Input: part model. Units: mm. Frame: model coordinates. Face numbers are marked on the shaded views. Coordinates: 2 decimals unless noted, no trailing zeros. Write each loop counter-clockwise with the first axis right and the second up, starting at its lowest first coordinate (ties: lowest second). Pieces come first, ordered by that corner, then holes. Notation, with made-up numbers: (65.25, 18) - (105.25, 18) arc R21 cw to (105.25, 39) - close; hole circle Ø7 at (-0.75, 36). An arc over 180 degrees is marked (long way). One line per question, with ' | ' between items. Start each with the question number.
1) First-contact query: P1, Ø2, axis at x = 8.5, y = 5, coming from the -Z side; P2, Ø5, axis at x = -27, y = 3.5, coming from the +Z side; P3, Ø3.5, axis at x = -19.5, z = -16, coming from the -Y side. Flat tips, straight axial feed; report the tip coordinate or a pass-through.
2) Section query C-C on y = 4. Return loops of the section in (x, z).
3) Section query D-D on x = -16.5. Return loops of the section in (y, z).
4) Line query: line 1 (Z direction, x = 12, y = 3.25); line 2 (Y direction, x = 11.5, z = -16); line 3 (Z direction, x = 12.5, y = 7). Output: solid intervals per line, ascending.
5) Draft query along Z for the marked faces 1 and 2. Return one class per face: released by +Z, released by -Z, zero draft, split by the parting line, or undercut.
6) Section query A-A on x = 34.5. Return loops of the section in (y, z) (3 decimals), and give its area (3 significant figures).
7) Section query B-B on z = 0. Return loops of the section in (x, y).
Autodesk Inventor part; units mm, degrees
ref_plane "YZ Plane" through (0, 0, 0) normal (1, 0, 0) x (0, 1, 0)
ref_plane "XZ Plane" through (0, 0, 0) normal (0, 1, 0) x (-1, 0, 0)
ref_plane "XY Plane" through (0, 0, 0) normal (0, 0, 1) x (1, 0, 0)
sketch "Base Pattern" plane through (0, 0, 0) normal (0, 1, 0) x (-1, 0, 0)
  line L0 (50, 13.5) -> (-50, 13.5)
  line L1 (-50, 13.5) -> (-50, -13.5)
  line L2 (-50, -13.5) -> (50, -13.5)
  line L3 (50, -13.5) -> (50, 13.5)
  line L4 (50, 13.5) -> (-50, -13.5) construction
  line L5 (-50, 13.5) -> (50, -13.5) construction
  point P0 (0, 0)
  dimension "Length" = 100
  dimension "Base_Width" = 27
sketch "Slot Pattern Set-Out" plane through (0, 0, 0) normal (0, 1, 0) x (-1, 0, 0)
  line L0 (0, -25) -> (0, 25)
  line L1 (10.385, 2.115) -> (-10.385, 2.115)
  line L2 (-10.385, -2.115) -> (10.385, -2.115)
  arc A0 (10.385, -2.115) -> (10.385, 2.115) centre (10.385, 0) ccw
  arc A1 (-10.385, 2.115) -> (-10.385, -2.115) centre (-10.385, 0) ccw
  line L3 (32, 0) -> (-32, 0) construction
  line L4 (10.385, 0) -> (-10.385, 0) construction
  point P0 (0, 0)
  point P1 (0, 0)
  point P2 (0, 0)
  point P3 (0, 0)
  dimension "Slot_Length" = 20.77
  dimension "Slot_Dia" = 4.23
  dimension "Pattern_Length" = 64
extrude "Plate1" add sketch "Base Pattern" along normal blind 1
sketch "Sketch3" plane through (-50, 0, -12.5) normal (0, 0, -1) x (-1, 0, 0)
  line L0 (-100, 0) -> (0, 0)
  line L1 (0, 0) -> (0, 7.5)
  line L2 (0, 7.5) -> (-100, 7.5)
  line L3 (-100, 7.5) -> (-100, 0)
edge flange "Flange Side" height 7.5 angle 90 thickness 1 bend radius 1 thickness toward (0, 0, -1) relief tear relief width 1 relief depth 0.5 corner gap 1 corner form 0 edges at (0, 1, -13.5) (0, 1, 13.5) wall of the first edge with corners at (50, 0, -12.5) (-50, 0, -12.5) (-50, 7.5, -12.5) (50, 7.5, -12.5)
bend "Bend1"
corner "Corner1"
sketch "Sketch4" plane through (-50, 7.5, 13.5) normal (0, 1, 0) x (-1, 0, 0)
  line L0 (-100, 0) -> (0, 0)
  line L1 (0, 0) -> (0, 4)
  line L2 (0, 4) -> (-100, 4)
  line L3 (-100, 4) -> (-100, 0)
edge flange "Flange Nib" height 5 angle 90 thickness 1 bend radius 1 thickness toward (0, 1, 0) relief tear relief width 1 relief depth 0.5 corner gap 1 corner form 0 edges at (0, 7.5, 13.5) (0, 7.5, -13.5) wall of the first edge with corners at (50, 7.5, 13.5) (-50, 7.5, 13.5) (-50, 7.5, 17.5) (50, 7.5, 17.5)
bend "Bend2"
corner "Corner2"
extrude "Slot Cut-Out" cut sketch "Slot Pattern Set-Out" along normal blind 1
pattern_linear "Slot Pattern" count 2 spacing 36 along (1, 0, 0) of "Slot Cut-Out"
mirror "Slot Patern Mirror" about plane through (0, 0, 0) normal (1, 0, 0) of "Slot Cut-Out", "Slot Pattern"
equation "\"Slot_Length\" = Slot_Length_Effective"
equation "\"d28\" = Thickness"
equation "\"d30\" = 0.6 * Slots_Integer"
equation "\"d32\" = Slot_Spacing"
equation "\"d33\" = Thickness"
equation "\"d8\" = BendReliefWidth"
equation "\"d9\" = BendReliefDepth"
equation "\"d10\" = MinimumRemnant"
equation "\"d11\" = BendRadius"
equation "\"d12\" = Flange_Height"
equation "\"d14\" = BendRadius"
equation "\"d15\" = CornerReliefSize"
equation "\"d16\" = GapSize"
equation "\"d17\" = JacobiRadiusSize"
equation "\"d18\" = BendReliefWidth"
equation "\"d19\" = BendReliefDepth"
equation "\"d20\" = MinimumRemnant"
equation "\"d21\" = BendRadius"
equation "\"d22\" = Flange_Nib"
equation "\"d24\" = BendRadius"
equation "\"d25\" = CornerReliefSize"
equation "\"d26\" = GapSize"
equation "\"d27\" = JacobiRadiusSize"
equation "\"BendRadius\" = Thickness"
equation "\"BendReliefWidth\" = Thickness"
equation "\"BendReliefDepth\" = 0.5 * Thickness"
equation "\"CornerReliefSize\" = 4 * Thickness"
equation "\"MinimumRemnant\" = 2 * Thickness"
equation "\"TransitionRadius\" = BendRadius"
equation "\"JacobiRadiusSize\" = BendRadius"
equation "\"GapSize\" = Thickness"
equation "\"Flange_Height\" = 7.5"
equation "\"Slot_Spacing\" = 36"
equation "\"Flange_Nib\" = 5"
equation "\"Slot_Length_Tab\" = 25"
equation "\"Slot_Length_Effective\" = Slot_Length_Tab - Slot_Dia"
properties part number "DIN Rail (TS) 35mm Wide v1-01" material "Steel"
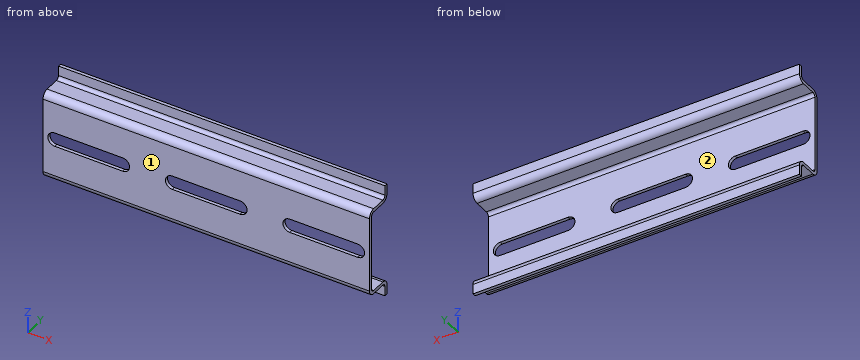
Answer key:
1) P1: z = -13.5 | P2: z = 13.5 | P3: y = 7.47
2) outline: (-50, -13.5) - (50, -13.5) - (50, -12.5) - (-50, -12.5) - close; (-50, 12.5) - (50, 12.5) - (50, 13.5) - (-50, 13.5) - close
3) outline: (0, -11.5) arc R2 ccw to (2, -13.5) - (6.5, -13.5) arc R1 cw to (7.5, -14.5) - (7.5, -17.5) - (8.5, -17.5) - (8.5, -14.5) arc R2 ccw to (6.5, -12.5) - (2, -12.5) arc R1 cw to (1, -11.5) - (1, 11.5) arc R1 cw to (2, 12.5) - (6.5, 12.5) arc R2 ccw to (8.5, 14.5) - (8.5, 17.5) - (7.5, 17.5) - (7.5, 14.5) arc R1 cw to (6.5, 13.5) - (2, 13.5) arc R2 ccw to (0, 11.5) - close
4) line 1: -13.5 to -12.5, 12.5 to 13.5 | line 2: 7.5 to 8.5 | line 3: -13.63 to -12.56, 12.56 to 13.63
5) face 1: zero draft | face 2: undercut
6) outline: (0, -11.5) arc R2 ccw to (2, -13.5) - (6.5, -13.5) arc R1 cw to (7.5, -14.5) - (7.5, -17.5) - (8.5, -17.5) - (8.5, -14.5) arc R2 ccw to (6.5, -12.5) - (2, -12.5) arc R1 cw to (1, -11.5) - (1, -2.115) - (0, -2.115) - close; (0, 2.115) - (1, 2.115) - (1, 11.5) arc R1 cw to (2, 12.5) - (6.5, 12.5) arc R2 ccw to (8.5, 14.5) - (8.5, 17.5) - (7.5, 17.5) - (7.5, 14.5) arc R1 cw to (6.5, 13.5) - (2, 13.5) arc R2 ccw to (0, 11.5) - close | area: 43.2 mm²
7) outline: (-50, 0) - (-48.5, 0) - (-48.5, 1) - (-50, 1) - close; (-23.5, 0) - (-12.5, 0) - (-12.5, 1) - (-23.5, 1) - close; (12.5, 0) - (23.5, 0) - (23.5, 1) - (12.5, 1) - close; (48.5, 0) - (50, 0) - (50, 1) - (48.5, 1) - close
